Check sheet for the modelled part. Datum: model origin and axes. Units: mm. A direction names the side the tool comes from. Give positions to 0.01 mm unless a question says otherwise; leave off trailing zeros. Write each loop counter-clockwise with the first axis right and the second up, starting at its lowest first coordinate (ties: lowest second). Pieces come first, ordered by that corner, then holes. Notation, with made-up numbers: M 9,-19 L 23,-19 A13 cw 23,-8 Z; hole C 7.25,-18.5 d8. An arc over 180 degrees is marked long. Write item = value, one per line. Start each with the question number.
1) Scan lines: L1, parallel to X at y = 3.75, z = 11.5 (3 decimals); L2, parallel to Y at x = -48, z = 20; L3, parallel to X at y = 12.25, z = -3. Record each from-to range of solid material in increasing order.
2) Set-up check for faces 1 (the face through (0.59, 7.021, 18.845)), 2 (the face through (41.025, 8, 15)), 3 (the face through (47.249, 5.743, 19.61)): record each of +Z, -Z, +X, -X, +Y, -Y from which the full face is reachable in a straight line by a thin tool's end or side.
3) Gauge pin test, flat ends, axial feed: pin 1 (4.5 mm diameter, centred on y = 7.5, z = 20, fed in from +X); pin 2 (12 mm diameter, centred on x = -1, z = 2.5, fed in from -Y); pin 3 (6 mm diameter, centred on y = 7.5, z = 20, fed in from +X). Record the tip position at first contact, or that the pin passes through.
4) Sectioned sample at A-A, the plane y = 7.5. Count the separate pieces of the cut face and the enclosed holes in it, then the cut area to 3 significant figures.
5) Sectioned sample at B-B, the plane z = 14. Record the cut outline in (x, y) (3 decimals), then the cut area to 3 significant figures.
6) Sectioned sample at C-C, the plane z = 20. Record the cut outline in (x, y) (3 decimals), then the cut area to 3 significant figures.
7) Sectioned sample at D-D, the plane x = 4. Record the cut outline in (y, z), then the cut area to 3 significant figures.
8) Draft check along Y on faces 4 (the face through (-6, 7, 0)), 5 (the face through (-1, 0, -11)), 6 (the face through (-47.294, 5.743, 20.39)). Enter one of: pulls with the +Y half, pulls with the -Y half, needs draft (parallel to the pull), parting line crosses it, or undercut.
from build123d import *

# Parameters (mm, degrees)
SKETCH1_W                                       = 110
SKETCH1_H                                       = 50
SKETCH1_R                                       = 6
BOSS_EXTRUDE2_DEPTH                             = 15
CUT_EXTRUDE1_DEPTH                              = 24
CSK_FOR_M3_FLAT_HEAD_MACHINE_SCREW1_D           = 3.6
CSK_FOR_M3_FLAT_HEAD_MACHINE_SCREW1_DEPTH       = 13.886032024
CSK_FOR_M3_FLAT_HEAD_MACHINE_SCREW1_CSINK_D     = 6.3
CSK_FOR_M3_FLAT_HEAD_MACHINE_SCREW1_CSINK_ANGLE = 90
CSK_FOR_M3_FLAT_HEAD_MACHINE_SCREW1_TIP         = 1.081549114
CSK_FOR_M3_FLAT_HEAD_MACHINE_SCREW2_D           = 3.6
CSK_FOR_M3_FLAT_HEAD_MACHINE_SCREW2_DEPTH       = 13.975
CSK_FOR_M3_FLAT_HEAD_MACHINE_SCREW2_CSINK_D     = 6.3
CSK_FOR_M3_FLAT_HEAD_MACHINE_SCREW2_CSINK_ANGLE = 90
CSK_FOR_M3_FLAT_HEAD_MACHINE_SCREW2_TIP         = 1.081549114
TAP_DRILL_FOR_M3X0_5_TAP1_D                     = 2.5


with BuildPart() as part:
    # Sketch1 → Boss-Extrude2 (new body)
    with BuildSketch(Plane(origin=(0, 0, 0), x_dir=(1, 0, 0), z_dir=(0, 1, 0))):
        Rectangle(SKETCH1_W, SKETCH1_H)
        Circle(SKETCH1_R, mode=Mode.SUBTRACT)
    extrude(amount=BOSS_EXTRUDE2_DEPTH)

    # Sketch2 → Cut-Extrude1 (cut)
    with BuildSketch(Plane(origin=(0, 15, 0), x_dir=(1, 0, 0), z_dir=(0, 1, 0))):
        with BuildLine():
            Line((-41.113967976, -25), (-38.886032024, -25))
            Line((-38.886032024, -25), (-38.886032024, -3.938852881))
            ThreePointArc((-38.886032024, -3.938852881), (-40, 4.106913882), (-41.113967976, -3.938852881))
            Line((-41.113967976, -3.938852881), (-41.113967976, -25))
        make_face()
        with BuildLine():
            Line((38.975, -25), (41.025, -25))
            Line((41.025, -25), (41.025, -3.962894048))
            ThreePointArc((41.025, -3.962894048), (40, 4.106913882), (38.975, -3.962894048))
            Line((38.975, -3.962894048), (38.975, -25))
        make_face()
    extrude(amount=-CUT_EXTRUDE1_DEPTH, mode=Mode.SUBTRACT)

    # CSK for M3 Flat Head Machine Screw1
    with Locations(Plane.ZY.offset(55)):
        with Locations((20, 7.5)):
            CounterSinkHole(CSK_FOR_M3_FLAT_HEAD_MACHINE_SCREW1_D / 2, CSK_FOR_M3_FLAT_HEAD_MACHINE_SCREW1_CSINK_D / 2, depth=CSK_FOR_M3_FLAT_HEAD_MACHINE_SCREW1_DEPTH, counter_sink_angle=CSK_FOR_M3_FLAT_HEAD_MACHINE_SCREW1_CSINK_ANGLE)
            with Locations((0, 0, -(CSK_FOR_M3_FLAT_HEAD_MACHINE_SCREW1_DEPTH + CSK_FOR_M3_FLAT_HEAD_MACHINE_SCREW1_TIP / 2))):  # 118° drill point
                Cone(0, CSK_FOR_M3_FLAT_HEAD_MACHINE_SCREW1_D / 2, CSK_FOR_M3_FLAT_HEAD_MACHINE_SCREW1_TIP, mode=Mode.SUBTRACT)

    # CSK for M3 Flat Head Machine Screw2
    with Locations(Plane(origin=(55, 0, 0), x_dir=(0, 0, -1), z_dir=(1, 0, 0))):
        with Locations((-20, 7.5)):
            CounterSinkHole(CSK_FOR_M3_FLAT_HEAD_MACHINE_SCREW2_D / 2, CSK_FOR_M3_FLAT_HEAD_MACHINE_SCREW2_CSINK_D / 2, depth=CSK_FOR_M3_FLAT_HEAD_MACHINE_SCREW2_DEPTH, counter_sink_angle=CSK_FOR_M3_FLAT_HEAD_MACHINE_SCREW2_CSINK_ANGLE)
            with Locations((0, 0, -(CSK_FOR_M3_FLAT_HEAD_MACHINE_SCREW2_DEPTH + CSK_FOR_M3_FLAT_HEAD_MACHINE_SCREW2_TIP / 2))):  # 118° drill point
                Cone(0, CSK_FOR_M3_FLAT_HEAD_MACHINE_SCREW2_D / 2, CSK_FOR_M3_FLAT_HEAD_MACHINE_SCREW2_TIP, mode=Mode.SUBTRACT)

    # Tap Drill for M3x0.5 Tap1 (through all)
    with Locations(Plane.ZY.offset(38.886032024)):
        with Locations((20, 7.5)):
            Hole(TAP_DRILL_FOR_M3X0_5_TAP1_D / 2)


solid = part.part
Data:
q1.L1 = -55 to -41.114, -38.886 to 38.975, 41.025 to 55
q1.L2 = 0 to 5.7, 9.3 to 15
q1.L3 = -55 to -42.8, -37.2 to -5.2, 5.2 to 37.2, 42.8 to 55
q2.face_1 = +X, -X
q2.face_2 = +Z, +Y, -Y
q2.face_3 = +X
q3.pin_1 = 54.1
q3.pin_2 = 0
q3.pin_3 = 54.85
q4.separate_pieces = 4
q4.enclosed_holes = 1
q4.area = 4,890 mm2
q5.outline = M -55,0 L -41.114,0 L -41.114,15 L -55,15 Z; M -38.886,0 L 38.975,0 L 38.975,15 L -38.886,15 Z; M 41.025,0 L 55,0 L 55,15 L 41.025,15 Z
q5.area = 1,590 mm2
q6.outline = M -55,0 L -41.114,0 L -41.114,5.7 L -53.65,5.7 L -55,4.35 Z; M -55,10.65 L -53.65,9.3 L -41.114,9.3 L -41.114,15 L -55,15 Z; M -38.886,0 L 38.975,0 L 38.975,6.25 L -38.886,6.25 Z; M -38.886,8.75 L 38.975,8.75 L 38.975,15 L -38.886,15 Z; M 41.025,0 L 55,0 L 55,4.35 L 53.65,5.7 L 41.025,5.7 Z; M 41.025,9.3 L 53.65,9.3 L 55,10.65 L 55,15 L 41.025,15 Z
q6.area = 1,290 mm2
q7.outline = M 0,-25 L 15,-25 L 15,-4.47 L 0,-4.47 Z; M 0,4.47 L 15,4.47 L 15,25 L 0,25 Z; hole C 7.5,20 d2.5
q7.area = 611 mm2
q8.face_4 = needs draft
q8.face_5 = pulls with the -Y half
q8.face_6 = undercut
